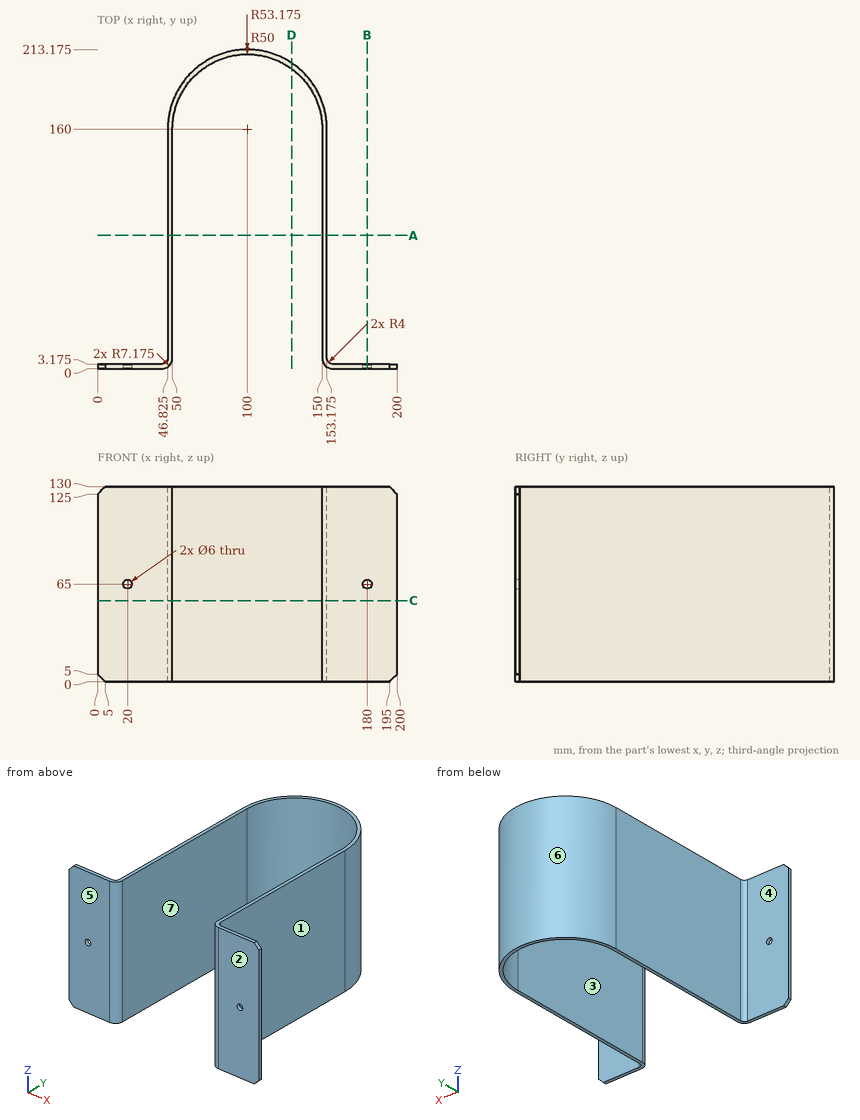
Geometry: see drawing. Coordinates: mm, zero at the bounding-box minimum. A direction names the side the tool comes from. Give positions to 0.01 mm unless a question says otherwise; leave off trailing zeros. Loops run counter-clockwise (first coordinate to the right, second up) from the corner with the lowest first, then second, coordinate; pieces in that order, holes last. Notation, with made-up numbers: (42, 11) -> (63, 11) arc R30 cw to (63, 35) -> close; hole circle Ø7 at (-40, -23.75). An arc over 180 degrees is marked (long way). Use CSV: the item, a comma, the result in double quotes.
(1) Access query for the marked faces 1, 2, 3 and 4. Directions: +Z, -Z, +X, -X, +Y, -Y. A direction counts if a zero-diameter tool reaches every point of the face in a straight line with its end or side. Return the directions, or none.
From the geometry:
face 1,"+Z, -Z, +X, +Y"
face 2,"+Z, -Z, +X, -X, -Y"
face 3,"+Z, -Z, -Y"
face 4,"+Z, -Z, -X, +Y"
(2) Cut plane C-C (z = 54). Output: boundary loops of the cut face in (x, y) (3 decimals), plus the area to 3 significant figures.
From the geometry:
outline,"(0, 0) -> (42.825, 0) arc R7.175 ccw to (50, 7.175) -> (50, 160) arc R50 cw to (150, 160) -> (150, 7.175) arc R7.175 ccw to (157.175, 0) -> (200, 0) -> (200, 3.175) -> (157.175, 3.175) arc R4 cw to (153.175, 7.175) -> (153.175, 160) arc R53.175 ccw to (46.825, 160) -> (46.825, 7.175) arc R4 cw to (42.825, 3.175) -> (0, 3.175) -> close"
area,"1,810 mm^2"
(3) Cut plane B-B (x = 180). Output: boundary loops of the cut face in (y, z) (3 decimals).
From the geometry:
outline,"(0, 0) -> (3.175, 0) -> (3.175, 62) -> (0, 62) -> close; (0, 68) -> (3.175, 68) -> (3.175, 130) -> (0, 130) -> close"
(4) First-contact query: P1, Ø4, axis at y = 29, z = 16.5, coming from the -X side (3 decimals); P2, Ø6, axis at x = 151.5, z = 68, coming from the -Y side; P3, Ø13, axis at x = 11, z = 60.5, coming from the +Y side (3 decimals). Flat tips, straight axial feed; report the tip coordinate or a pass-through.
From the geometry:
P1,"x = 46.825"
P2,"y = 0.52"
P3,"y = 3.175"
(5) Ray query, line 1 along X through (y, z) = (1.8, 65); line 2 along X through (y, z) = (0.8, 65); line 3 along Z through (x, y) = (20, 1.65). Return the intervals inside material, ascending. Write a range as [from, to].
From the geometry:
line 1,"[0, 17], [23, 47.58], [152.42, 177], [183, 200]"
line 2,"[0, 17], [23, 46.12], [153.88, 177], [183, 200]"
line 3,"[0, 62], [68, 130]"
(6) Cut plane D-D (x = 129.5). Output: boundary loops of the cut face in (y, z), plus the area to 3 significant figures.
From the geometry:
outline,"(200.37, 0) -> (204.24, 0) -> (204.24, 130) -> (200.37, 130) -> close"
area,"503 mm^2"
(7) Pull-direction query (X, two-part tool) for the marked faces 5, 6 and 7; classes: released by +X, released by -X, zero draft, split by the parting line, or undercut.
From the geometry:
face 5,"zero draft"
face 6,"split by the parting line"
face 7,"undercut"
(8) Cut plane A-A (y = 89). Output: boundary loops of the cut face in (x, z) (3 decimals), plus the area to 4 significant figures.
From the geometry:
outline,"(46.825, 0) -> (50, 0) -> (50, 130) -> (46.825, 130) -> close; (150, 0) -> (153.175, 0) -> (153.175, 130) -> (150, 130) -> close"
area,"825.5 mm^2"
